Here's how the part is built. I have some questions about the finished solid (model axes, mm). Coordinates: 2 decimals unless noted, no trailing zeros. Write each loop counter-clockwise with the first axis right and the second up, starting at its lowest first coordinate (ties: lowest second). Pieces come first, ordered by that corner, then holes.
Item 1: If we section it at B-B (z = 5.5): Please give me the cut outline in (x, y) (1 decimal).
Item 2: If I drill on line 1 (Y direction, x = 2.75, z = 1); line 2 (Y direction, x = 0.75, z = 5.5); line 3 (X direction, y = 2, z = 2.25), over which ranges is the centre line in solid material (lowest first)?
Item 3: If we section it at A-A (z = 1.25): Please give me the cut outline in (x, y).
Item 4: I'm going to push flat-ended pins straight in: pin 1 Ø1 at (x, z) = (1.5, 1) entering from -Y; pin 2 Ø2 at (y, z) = (3, 1.5) entering from +X; pin 3 Ø5 at (x, y) = (-3, 2.5) entering from +Z. Where does each tip first touch, or does it pass through?
from build123d import *

# Parameters (mm, degrees)
F0_R        = 3.89
F1_DEPTH    = 3
F2_R        = 4.585
F2_R_2      = 3.89
F5_DEPTH    = 1
F5_FACE_R   = 4.585
F4_R        = 2
F7_R        = 2.5
F8_S5_R     = 3.89
F8_T6_DEPTH = 8


# Not quite as in the source:
# - a fillet or chamfer that OpenCascade refuses, or shapes differently, is made with other operations: its cross-section is extruded or revolved along the edge and cut away or added


with BuildPart() as f1:
    # F0 (on Top) → F1 (new body)
    with BuildSketch(Plane.XY):
        Circle(F0_R)
    extrude(amount=F1_DEPTH)

    # F2 (on face) → F5 (join)
    with BuildSketch(Plane.XY.offset(3)):
        Circle(F2_R)
        Circle(F2_R_2, mode=Mode.SUBTRACT)
        Circle(F2_R_2)
    extrude(amount=F5_DEPTH)

    # F5_face (on face) → F6 section 0
    with BuildSketch(Plane.XY.offset(4)):
        Circle(F5_FACE_R)
    # F4 (on offset) → F6 section 1
    with BuildSketch(Plane.XY.offset(7)):
        Circle(F4_R)
    loft()

    # F7
    f7_edges = [f1.edges().sort_by_distance(p)[0] for p in [
        (-2, 0, 7),
    ]]
    fillet(f7_edges, radius=F7_R)

    # F8: chamfer of 0.7 on 1 edges, made by hand


with BuildPart() as f8_tool2:
    # F8_s3 → F8_t4 (revolve)
    with BuildSketch(Plane.XZ):
        Polygon((4.585, 3.7), (3.885, 3), (4.585, 3), align=None)
    revolve(axis=Axis((0, 0, 3), (0, 0, 1)))

    # F8_s5 → F8_t6 (cut, symmetric)
    with BuildSketch(Plane.XY.offset(3.4)):
        Circle(F8_S5_R)
    extrude(amount=F8_T6_DEPTH, both=True, mode=Mode.SUBTRACT)


with BuildPart() as f1_1:
    add(f1.part)

    # F8_t1: cut F8_tool2
    add(f8_tool2.part, mode=Mode.SUBTRACT)


solid = f1_1.part
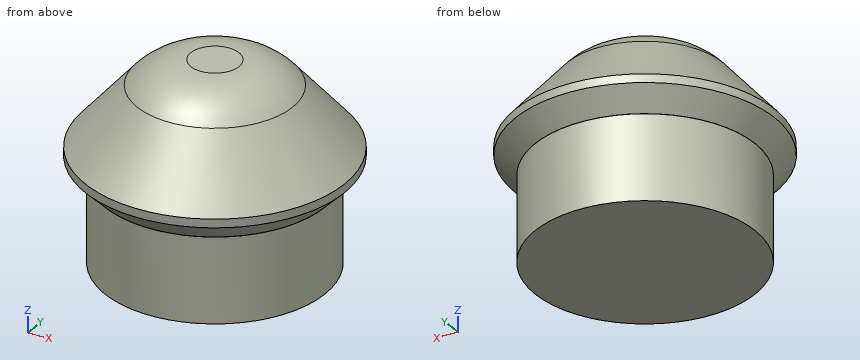
Answer list:
1. outline: circle Ø6.6 at (0, 0)
2. line 1: y = -2.75 to 2.75
2. line 2: y = -3.21 to 3.21
2. line 3: x = -3.34 to 3.34
3. outline: circle Ø7.78 at (0, 0)
4. pin 1: stops at y = -3.76
4. pin 2: stops at x = 3.34
4. pin 3: stops at z = 6.94
